```python
from build123d import *

# Parameters (mm, degrees)
ESBO_O2_R                  = 2.5
CORTE_EXTRUS_O1_DEPTH      = 19.629009636
ESBO_O4_R                  = 1
CORTE_EXTRUS_O2_DEPTH      = 7
CORTE_EXTRUS_O3_DEPTH      = 19.629009636
CORTE_EXTRUS_O3_DEPTH_BACK = 19.629009636
ESBO_O5_R                  = 1.5
FILETE1_R                  = 0.2


with BuildPart() as part:
    # Esboço1 → Revolução1 (revolve)
    with BuildSketch(Plane(origin=(0, 0, 0), x_dir=(0, 0, -1), z_dir=(1, 0, 0)), mode=Mode.PRIVATE) as revolu_o1_sk:
        with BuildLine():
            Line((0, 7), (0, 3.9))
            ThreePointArc((0, 3.9), (0.029289322, 3.829289322), (0.1, 3.8))
            Line((0.1, 3.8), (0.4, 3.8))
            Line((0.4, 3.8), (0, 3.5))
            Line((0, 3.5), (0, 0))
            Line((0, 0), (14.8, 0))
            Line((14.8, 0), (14.8, 3.854253969))
            Line((14.8, 3.854253969), (14.3, 4.354253969))
            Line((14.3, 4.354253969), (13.977126984, 4.354253969))
            Line((13.977126984, 4.354253969), (13.977126984, 6.354253969))
            Line((13.977126984, 6.354253969), (14.8, 8))
            Line((14.8, 8), (13.8, 8))
            Line((13.8, 8), (13, 6.4))
            Line((13, 6.4), (6, 6.4))
            Line((6, 6.4), (6, 7))
            Line((6, 7), (5.5, 8))
            Line((5.5, 8), (0.5, 8))
            Line((0.5, 8), (0, 7))
        make_face()
    revolve(revolu_o1_sk.sketch.rotate(Axis((0, 0, 0), (0, 0, -1)), 90), axis=Axis((0, 0, 0), (0, 0, -1)))

    # Esboço2 → Corte-extrusão1 (cut, through all)
    with BuildSketch(Plane(origin=(0, 0, -14.8), x_dir=(-1, 0, 0), z_dir=(0, 0, -1))):
        Circle(ESBO_O2_R)
    extrude(amount=-CORTE_EXTRUS_O1_DEPTH, mode=Mode.SUBTRACT)

    # Esboço4 → Corte-extrusão2 (cut)
    with BuildSketch(Plane(origin=(0, 0, -6), x_dir=(-1, 0, 0), z_dir=(0, 0, -1))):
        with Locations((0, 6.4)):
            Circle(ESBO_O4_R)
        with Locations((2.77685593, 5.766200755)):
            Circle(ESBO_O4_R)
        with Locations((5.003721488, 3.990334732)):
            Circle(ESBO_O4_R)
        with Locations((6.239538638, 1.424133977)):
            Circle(ESBO_O4_R)
        with Locations((6.239538638, -1.424133977)):
            Circle(ESBO_O4_R)
        with Locations((5.003721488, -3.990334732)):
            Circle(ESBO_O4_R)
        with Locations((2.77685593, -5.766200755)):
            Circle(ESBO_O4_R)
        with Locations((0, -6.4)):
            Circle(ESBO_O4_R)
        with Locations((-2.77685593, -5.766200755)):
            Circle(ESBO_O4_R)
        with Locations((-5.003721488, -3.990334732)):
            Circle(ESBO_O4_R)
        with Locations((-6.239538638, -1.424133977)):
            Circle(ESBO_O4_R)
        with Locations((-6.239538638, 1.424133977)):
            Circle(ESBO_O4_R)
        with Locations((-5.003721488, 3.990334732)):
            Circle(ESBO_O4_R)
        with Locations((-2.77685593, 5.766200755)):
            Circle(ESBO_O4_R)
    extrude(amount=CORTE_EXTRUS_O2_DEPTH, mode=Mode.SUBTRACT)

    # Esboço5 → Corte-extrusão3 (cut, two sides: drawn at the far end of the back side and taken through both)
    with BuildSketch(Plane(origin=(0, 0, 0), x_dir=(0, 0, -1), z_dir=(1, 0, 0)).offset(-CORTE_EXTRUS_O3_DEPTH_BACK)):
        with Locations(Location((3, 0, 0), (0, 0, 180))):
            Circle(ESBO_O5_R)
    extrude(amount=CORTE_EXTRUS_O3_DEPTH + CORTE_EXTRUS_O3_DEPTH_BACK, mode=Mode.SUBTRACT)

    # Filete1
    filete1_edges = [part.edges().sort_by_distance(p)[0] for p in [
        (7.858116823, 1.5, -3),
        (-8, 0, -4.5),
    ]]
    fillet(filete1_edges, radius=FILETE1_R)


solid = part.part
```
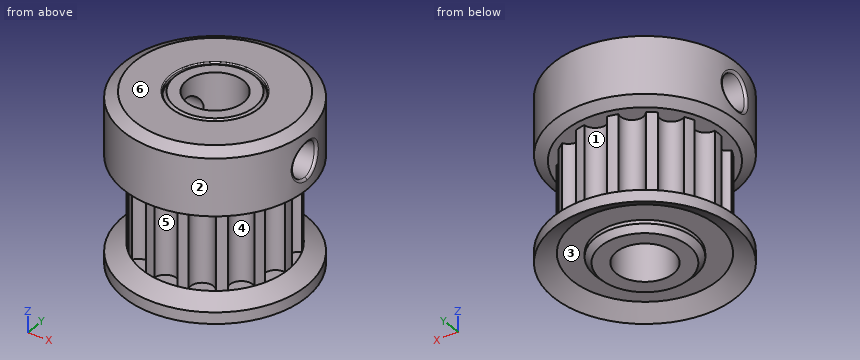
Read the model definition and answer for the solid it produces. Units are mm, in the model's axes. Face numbers are marked on the shaded views. A direction names the side the tool comes from. Round coordinates to 2 decimals unless told otherwise and drop trailing zeros. Answer in a Markdown table with one row per item. Add a question column.
1) Given P1, Ø1, axis at x = 2.5, y = 3, coming from the +Z side; P2, Ø4, axis at y = 3.5, z = -9, coming from the +X side; P3, Ø5, axis at y = 4, z = -9.5, coming from the -X side; P4, Ø2.5, axis at y = 0, z = -3, coming from the -X side, each flat-ended and moving along its own axis, determine where each tip first touches the part or whether it passes through.
2) Determine the mould class of the marked faces 1, 2 and 3 for opening direction Y: pulls with the +Y half, pulls with the -Y half, needs draft (parallel to the pull), parting line crosses it, or undercut.
3) Consider line 1 (Y direction, x = 0, z = -7.5); line 2 (Z direction, x = 0, y = -6); line 3 (Y direction, x = 2, z = -2.5). Determine where each line is inside the solid, lowest interval first.
4) Which of the six approach directions +Z, -Z, +X, -X, +Y, -Y give full straight-line access (tool end or side, diameter ignored) to the marked faces 4, 5 and 6?
Findings below:
| question | item | result |
|---|---|---|
| 1 | P1 | z = 0 |
| 1 | P2 | x = 5.94 |
| 1 | P3 | x = -5.94 |
| 1 | P4 | through |
| 2 | face 1 | pulls with the +Y half |
| 2 | face 2 | parting line crosses it |
| 2 | face 3 | undercut |
| 3 | line 1 | -5.4 to -2.5, 2.5 to 5.4 |
| 3 | line 2 | -13.98 to -13, -6 to 0 |
| 3 | line 3 | -7.75 to -1.5, 1.5 to 7.75 |
| 4 | face 4 | none |
| 4 | face 5 | -Y |
| 4 | face 6 | +Z, +X, -X, +Y, -Y |
